Could you check a few things on this model? Use its own coordinates, in mm. A direction names the side the tool comes from. Coordinates: 2 decimals unless noted, no trailing zeros. Loops run counter-clockwise (first coordinate to the right, second up) from the corner with the lowest first, then second, coordinate; pieces in that order, holes last.
1) Imagine slicing it at B-B on x = 13. Please give me the cut outline in (y, z).
2) For faces 1 (the face through (30.16, -30.85, 30.63)), 2 (the face through (1, -24, 4)), 3 (the face through (-6.993, -29, 4)), 4 (the face through (33.785, -37, 27)), which set-ups out of +Z, -Z, +X, -X, +Y, -Y let a thin tool reach every point of the face, with its end or its side?
3) Imagine slicing it at C-C on z = 0. Please give me the cut outline in (x, y).
4) Thinking about a two-plate mould opening in X: for faces 5 (the face through (11, -22, 28.344)), 6 (the face through (19.554, -15.002, 30.562)), 7 (the face through (34.641, -36.704, 21.114)), 8 (the face through (-11.215, -37, 27)), which applies, released by +X, released by -X, zero draft, split by the parting line, or undercut?
5) Imagine slicing it at A-A on y = -13.5. Please give me the cut outline in (x, z), plus the area to 3 significant figures.
6) Will these pins go through, and if not, where does the flat tip stop? P1, Ø1.5, axis at y = -34.5, z = -3.5, coming from the -X side; P2, Ø4, axis at y = -37.5, z = 27.5, coming from the -X side; P3, Ø5, axis at y = -30.5, z = 2.5, coming from the -X side; P4, Ø6, axis at x = 14.79, y = -13.5, coming from the -Z side.
7) Imagine slicing it at D-D on x = 3. Please give me the cut outline in (y, z), plus the area to 3 significant figures.
8) If I drill on line 1 along Z through (x, y) = (25.5, -25); line 2 along Y through (x, z) = (11, -1); line 3 along X through (y, z) = (-9, -4.5), over which ranges is the centre line in solid material (lowest first)?
```python
from build123d import *

# Parameters (mm, degrees)
F0_R      = 5.25
F0_R_2    = 6
F1_DEPTH  = 40
F2_W      = 50
F2_H      = 29.5
F3_DEPTH  = 100
F4_DEPTH  = 100
F5_R      = 5
F6_DEPTH  = 50
F8_DEPTH  = 15
F10_DEPTH = 15
F11_W     = 15
F11_H     = 11
F12_DEPTH = 9.5


with BuildPart() as f1:
    # F0 (on Front) → F1 (new body)
    with BuildSketch(Plane.XZ):
        with BuildLine():
            Line((30.785211, 32.843663), (-8.214789, 32.843663))
            ThreePointArc((-8.214789, 32.843663), (-10.336109, 31.964984), (-11.214789, 29.843663))
            Line((-11.214789, 29.843663), (-11.214789, 25.048589))
            ThreePointArc((-11.214789, 25.048589), (-12.544869, 21.652755), (-15.827465, 20.063614))
            ThreePointArc((-15.827465, 20.063614), (-24.791107, 12.366478), (-20.160798, 1.496657))
            ThreePointArc((-20.160798, 1.496657), (-18.369104, -0.328989), (-17.714789, -2.801847))
            Line((-17.714789, -2.801847), (-17.714789, -4.156337))
            ThreePointArc((-17.714789, -4.156337), (-16.836109, -6.277657), (-14.714789, -7.156337))
            Line((-14.714789, -7.156337), (30.785211, -7.156337))
            ThreePointArc((30.785211, -7.156337), (32.906531, -6.277657), (33.785211, -4.156337))
            Line((33.785211, -4.156337), (33.785211, -3.723625))
            ThreePointArc((33.785211, -3.723625), (34.618075, -0.960478), (36.839202, 0.882138))
            ThreePointArc((36.839202, 0.882138), (42.947184, 10.093663), (36.839202, 19.305188))
            ThreePointArc((36.839202, 19.305188), (34.618075, 21.147805), (33.785211, 23.910951))
            Line((33.785211, 23.910951), (33.785211, 29.843663))
            ThreePointArc((33.785211, 29.843663), (32.906531, 31.964984), (30.785211, 32.843663))
        make_face()
        with Locations((-15.052816, 10.093663)):
            Circle(F0_R, mode=Mode.SUBTRACT)
        with Locations((32.947184, 10.093663)):
            Circle(F0_R, mode=Mode.SUBTRACT)
        with Locations((12.493362, 19.468693)):
            Circle(F0_R_2, mode=Mode.SUBTRACT)
    extrude(amount=F1_DEPTH)

    # F2 (on Right) → F3 (cut)
    with BuildSketch(Plane.YZ):
        with Locations((-8.5, 13.593663)):
            Rectangle(F2_W, F2_H)
    extrude(amount=-F3_DEPTH, mode=Mode.SUBTRACT)

    # F2 (on Right) → F4 (cut)
    with BuildSketch(Plane.YZ):
        with Locations((-8.5, 13.593663)):
            Rectangle(F2_W, F2_H)
    extrude(amount=F4_DEPTH, mode=Mode.SUBTRACT)

    # F5 (on face) → F6 (cut)
    with BuildSketch(Plane(origin=(0, 0, -7.156337), x_dir=(1, 0, 0), z_dir=(0, 0, -1))):
        with Locations((14.785211, 13.5)):
            Circle(F5_R)
    extrude(amount=-F6_DEPTH, mode=Mode.SUBTRACT)

    # F7 (on face) → F8 (cut)
    with BuildSketch(Plane(origin=(0, 0, -7.156337), x_dir=(1, 0, 0), z_dir=(0, 0, -1))):
        with BuildLine():
            ThreePointArc((25.095301, 8.405686), (16.964946, 2.208465), (7.112094, 4.93418))
            Line((7.112094, 4.93418), (-14.714789, 24.486333))
            Line((-14.714789, 24.486333), (-14.714789, 0))
            Line((-14.714789, 0), (30.785211, 0))
            Line((30.785211, 0), (30.785211, 19.921168))
            Line((30.785211, 19.921168), (25.095301, 8.405686))
        make_face()
        Polygon((-14.714789, 0), (-14.714789, 24.486333), (-18.07907, 27.5), (-24.334732, 27.5), (-24.334732, -4.176865), (44.914905, -4.176865), (44.914905, 27.5), (34.529984, 27.5), (30.785211, 19.921168), (30.785211, 0), align=None)
    extrude(amount=-F8_DEPTH, mode=Mode.SUBTRACT)

    # F9 (on face) → F10 (cut)
    with BuildSketch(Plane.XY.offset(32.843663)):
        with BuildLine():
            ThreePointArc((6.11086, -8.524496), (16.017743, -3.576248), (24.413154, -10.797646))
            Line((24.413154, -10.797646), (29.761066, -29.851177))
            ThreePointArc((29.761066, -29.851177), (30.168378, -30.86249), (30.785211, -31.761475))
            Line((30.785211, -31.761475), (30.785211, 0))
            Line((30.785211, 0), (-8.214789, 0))
            Line((-8.214789, 0), (-8.214789, -32.575799))
            ThreePointArc((-8.214789, -32.575799), (-7.408155, -31.859936), (-6.773794, -30.987752))
            Line((-6.773794, -30.987752), (6.11086, -8.524496))
        make_face()
        with BuildLine():
            Line((30.785211, 0), (30.785211, -31.761475))
            ThreePointArc((30.785211, -31.761475), (32.490256, -33.044633), (34.575037, -33.5))
            Line((34.575037, -33.5), (55.997241, -33.5))
            Line((55.997241, -33.5), (49.117599, 6.79242))
            Line((49.117599, 6.79242), (-12.63734, 6.79242))
            Line((-12.63734, 6.79242), (-31.90035, -33.5))
            Line((-31.90035, -33.5), (-11.110969, -33.5))
            ThreePointArc((-11.110969, -33.5), (-9.590936, -33.26335), (-8.214789, -32.575799))
            Line((-8.214789, -32.575799), (-8.214789, 0))
            Line((-8.214789, 0), (30.785211, 0))
        make_face()
    extrude(amount=-F10_DEPTH, mode=Mode.SUBTRACT)

    # F11 (on face) → F12 (join)
    with BuildSketch(Plane(origin=(0, -33.5, 0), x_dir=(-1, 0, 0), z_dir=(0, 1, 0))):
        with Locations((-0.506683, 4.343663)):
            Rectangle(F11_W, F11_H)
    extrude(amount=F12_DEPTH)


solid = f1.part
```
Filled in:
1. outline: (-40, -7.16) - (-18.17, -7.16) - (-18.17, -1.16) - (-33.5, -1.16) - (-33.5, 13.49) - (-40, 13.49) - close; (-40, 25.45) - (-33.5, 25.45) - (-33.5, 28.34) - (-18.17, 28.34) - (-18.17, 32.84) - (-40, 32.84) - close; (-8.83, -7.16) - (-2.14, -7.16) - (-2.14, -1.16) - (-8.83, -1.16) - close; (-8.83, 28.34) - (-3.66, 28.34) - (-3.66, 32.84) - (-8.83, 32.84) - close
2. face 1: +Z, +X, +Y
2. face 2: +X, -X, +Y
2. face 3: -X, +Y
2. face 4: +Z, +X, +Y, -Y
3. outline: (-18.57, -40) - (35.45, -40) - (35.45, -33.5) - (8.01, -33.5) - (8.01, -24) - (-6.99, -24) - (-6.99, -33.5) - (-18.57, -33.5) - close
4. face 5: zero draft
4. face 6: undercut
4. face 7: released by +X
4. face 8: released by -X
5. outline: (-2.45, -7.16) - (9.79, -7.16) - (9.79, -1.16) - (-2.45, -1.16) - close; (3.26, 28.34) - (9.79, 28.34) - (9.79, 32.84) - (3.26, 32.84) - close; (19.79, -7.16) - (27.61, -7.16) - (27.61, -1.16) - (19.79, -1.16) - close; (19.79, 28.34) - (25.17, 28.34) - (25.17, 32.84) - (19.79, 32.84) - close
5. area: 174 mm2
6. P1: stops at x = -17.72
6. P2: stops at x = -11.21
6. P3: stops at x = -6.99
6. P4: passes through
7. outline: (-40, -7.16) - (-8.62, -7.16) - (-8.62, -1.16) - (-24, -1.16) - (-24, 9.84) - (-33.5, 9.84) - (-33.5, 28.34) - (-13.95, 28.34) - (-13.95, 32.84) - (-40, 32.84) - close
7. area: 602 mm2
8. line 1: z = -7.16 to -1.16, 28.34 to 32.84
8. line 2: y = -40 to -33.5
8. line 3: x = 2.57 to 12.61, 16.96 to 25.39
